from build123d import *

# Parameters (mm, degrees)
BOSS_EXTRUDE1_OUTLINE_W   = 227.076
BOSS_EXTRUDE1_OUTLINE_H   = 508
BOSS_EXTRUDE1_OUTLINE_R   = 14.2875
BOSS_EXTRUDE1_OUTLINE_R_2 = 2.5527
BOSS_EXTRUDE1_OUTLINE_R_3 = 9.525
BOSS_EXTRUDE1_DEPTH       = 1.5875
F_8_CLEARANCE_HOLE1_D     = 4.9149
CHAMFER1_SIZE             = 127
BOSS_EXTRUDE2_DEPTH       = 1.5875


# Read off the part's stored shape, not the designer's step: Boss-Extrude1
with BuildPart() as part:
    # Boss-Extrude1 outline → Boss-Extrude1 (new body)
    with BuildSketch(Plane(origin=(0, 0, 0), x_dir=(0, 0, -1), z_dir=(1, 0, 0))):
        Rectangle(BOSS_EXTRUDE1_OUTLINE_W, BOSS_EXTRUDE1_OUTLINE_H)
        with Locations((43.688, -122.2375)):
            Circle(BOSS_EXTRUDE1_OUTLINE_R, mode=Mode.SUBTRACT)
        with Locations((25.727487758, -14.254307758)):
            Circle(BOSS_EXTRUDE1_OUTLINE_R_2, mode=Mode.SUBTRACT)
        with Locations((43.688, -32.21482)):
            Circle(BOSS_EXTRUDE1_OUTLINE_R_3, mode=Mode.SUBTRACT)
        with Locations((61.648512242, -50.175332242)):
            Circle(BOSS_EXTRUDE1_OUTLINE_R_2, mode=Mode.SUBTRACT)
        with Locations((43.688, 52.78628)):
            Circle(BOSS_EXTRUDE1_OUTLINE_R, mode=Mode.SUBTRACT)
    extrude(amount=BOSS_EXTRUDE1_DEPTH)

    # #8 Clearance Hole1 (through all)
    with Locations(Plane(origin=(1.5875, 0, 0), x_dir=(0, 0, -1), z_dir=(1, 0, 0))):
        with Locations((-74.877168, -237.687866)):
            Hole(F_8_CLEARANCE_HOLE1_D / 2)

    # Chamfer1
    chamfer1_edges = [part.edges().sort_by_distance(p)[0] for p in [
        (0.79375, 254, -113.538),
    ]]
    chamfer(chamfer1_edges, length=CHAMFER1_SIZE)

    # Sketch7 → Boss-Extrude2 (add, through all)
    with BuildSketch(Plane(origin=(1.5875, 0, 0), x_dir=(0, 0, -1), z_dir=(1, 0, 0))):
        Polygon((-113.538, 254), (-113.538, 280.815283382), (-13.462, 254), align=None)
    extrude(amount=-BOSS_EXTRUDE2_DEPTH)


solid = part.part
Check sheet for the modelled part. Datum: model origin and axes. Units: mm. Give positions to 0.01 mm unless a question says otherwise; leave off trailing zeros. Loops run counter-clockwise (first coordinate to the right, second up) from the corner with the lowest first, then second, coordinate; pieces in that order, holes last. Notation, with made-up numbers: M 29,-26 L 42,-26 A18 ccw 42,-15 Z; hole C -34.75,72.5 d11. An arc over 180 degrees is marked long. Return JSON: item names as keys, results as strings. Group by question number.
1. Thickness scan on L1, parallel to Y at x = 0.9, z = -44; L2, parallel to Y at x = 1.4, z = -40.5; L3, parallel to Z at x = 1.05, y = -123. Record the ranges inside material, lowest first.
2. Mould release check, pull along Y, two halves, no side actions. Record for faces 1 (the flat face through (1.588, 17, -2)), 2 (the cylindrical face through (0.783, -134.913, -50.281)), 3 (the cylindrical face through (0.783, -41.513, -41.623)), 4 (the flat face through (0.805, 267.595, 64.201)): released by +Y, released by -Y, zero draft, split by the parting line, or undercut.
3. Cross-section at C-C on z = 33.5. Record the boundary of the cut face in (x, y).
4. Cross-section at A-A on z = -47. Record the boundary of the cut face in (x, y).
5. Cross-section at B-B on x = 1.25. State how many separate pieces and enclosed holes the cut face has, plus the area to 3 significant figures.
6. Cross-section at D-D on y = 245. Record the boundary of the cut face in (x, z).
Return value:
{
 "1": {"L1": "-254 to -136.52, -107.95 to -41.73, -22.69 to 38.5, 67.07 to 196.54", "L2": "-254 to -136.16, -108.31 to -41.19, -23.24 to 38.86, 66.71 to 200.04", "L3": "-113.54 to -57.96, -29.42 to 113.54"},
 "2": {"face 1": "zero draft", "face 2": "undercut", "face 3": "undercut", "face 4": "released by +Y"},
 "3": {"outline": "M 0,-254 L 1.59,-254 L 1.59,259.37 L 0,259.37 Z"},
 "4": {"outline": "M 0,-254 L 1.59,-254 L 1.59,-136.14 L 0,-136.14 Z; M 0,-108.34 L 1.59,-108.34 L 1.59,-41.15 L 0,-41.15 Z; M 0,-23.28 L 1.59,-23.28 L 1.59,38.89 L 0,38.89 Z; M 0,66.68 L 1.59,66.68 L 1.59,193.54 L 0,193.54 Z"},
 "5": {"separate pieces": "1", "enclosed holes": "6", "area": "107,000 mm^2"},
 "6": {"outline": "M 0,4.46 L 1.59,4.46 L 1.59,113.54 L 0,113.54 Z"}
}
